Verification items for the finished model (mm, model axes). A direction names the side the tool comes from. Round coordinates to 2 decimals unless told otherwise and drop trailing zeros. Write each loop counter-clockwise with the first axis right and the second up, starting at its lowest first coordinate (ties: lowest second). Pieces come first, ordered by that corner, then holes. Notation, with made-up numbers: (41, -32.5) - (46, -32.5) arc R29 ccw to (46, -6.5) - close; hole circle Ø5 at (44, 28). An arc over 180 degrees is marked (long way). Answer as a JSON object with one key per item and string values.
```python
from build123d import *

# Parameters (mm, degrees)
IZIM1_R                     = 2
IZIM1_R_2                   = 90
Y_KSEKLIK_EKSTR_ZYON1_DEPTH = 3
FILLET1_R                   = 5


with BuildPart() as part:
    # Çizim1 → Yükseklik-Ekstrüzyon1 (new body)
    with BuildSketch(Plane.XY):
        with BuildLine():
            ThreePointArc((81.317279836, -93.817279836), (68.980438262, -79.304237374), (85.290813588, -69.46565423))
            ThreePointArc((85.290813588, -69.46565423), (110, 0), (85.290813588, 69.46565423))
            ThreePointArc((85.290813588, 69.46565423), (68.980438262, 79.304237374), (81.317279836, 93.817279836))
            Line((81.317279836, 93.817279836), (89.317279836, 93.817279836))
            Line((89.317279836, 93.817279836), (89.317279836, 110))
            Line((89.317279836, 110), (-89.317279836, 110))
            Line((-89.317279836, 110), (-89.317279836, 93.817279836))
            Line((-89.317279836, 93.817279836), (-81.317279836, 93.817279836))
            ThreePointArc((-81.317279836, 93.817279836), (-68.980438262, 79.304237374), (-85.290813588, 69.46565423))
            ThreePointArc((-85.290813588, 69.46565423), (-110, 0), (-85.290813588, -69.46565423))
            ThreePointArc((-85.290813588, -69.46565423), (-68.980438262, -79.304237374), (-81.317279836, -93.817279836))
            Line((-81.317279836, -93.817279836), (-89.317279836, -93.817279836))
            Line((-89.317279836, -93.817279836), (-89.317279836, -110))
            Line((-89.317279836, -110), (89.317279836, -110))
            Line((89.317279836, -110), (89.317279836, -93.817279836))
            Line((89.317279836, -93.817279836), (81.317279836, -93.817279836))
        make_face()
        with Locations((-80.9, -101.317279836)):
            Circle(IZIM1_R, mode=Mode.SUBTRACT)
        with Locations((80.9, -101.317279836)):
            Circle(IZIM1_R, mode=Mode.SUBTRACT)
        Circle(IZIM1_R_2, mode=Mode.SUBTRACT)
        with Locations((64.9, 101.317279836)):
            Circle(IZIM1_R, mode=Mode.SUBTRACT)
        with Locations((80.9, 101.317279836)):
            Circle(IZIM1_R, mode=Mode.SUBTRACT)
        with Locations((-80.9, 101.317279836)):
            Circle(IZIM1_R, mode=Mode.SUBTRACT)
        with Locations((-64.9, 101.317279836)):
            Circle(IZIM1_R, mode=Mode.SUBTRACT)
        with Locations((64.9, -101.317279836)):
            Circle(IZIM1_R, mode=Mode.SUBTRACT)
        with Locations((-64.9, -101.317279836)):
            Circle(IZIM1_R, mode=Mode.SUBTRACT)
    extrude(amount=Y_KSEKLIK_EKSTR_ZYON1_DEPTH)

    # Fillet1
    fillet1_edges = [part.edges().sort_by_distance(p)[0] for p in [
        (89.317279836, -93.817279836, 1.5),
        (89.317279836, -110, 1.5),
        (-89.317279836, -110, 1.5),
        (-89.317279836, -93.817279836, 1.5),
        (-85.290813588, -69.46565423, 1.5),
        (-85.290813588, 69.46565423, 1.5),
        (-89.317279836, 93.817279836, 1.5),
        (-89.317279836, 110, 1.5),
        (89.317279836, 110, 1.5),
        (89.317279836, 93.817279836, 1.5),
        (85.290813588, 69.46565423, 1.5),
        (85.290813588, -69.46565423, 1.5),
    ]]
    fillet(fillet1_edges, radius=FILLET1_R)


solid = part.part
```
1. Cross-section at C-C (z = 2.15). Count the separate pieces of the cut face and the enclosed holes in it, plus the area to 3 significant figures.
Completed:
{"separate pieces": "1", "enclosed holes": "9", "area": "15,500 mm^2"}
2. Access from +Z, -Z, +X, -X, +Y, -Y to the whole of each face (thin tool, end or side, straight path). Record for faces 1 (the face through (-87.814, 108.574, 1.521)), 2 (the face through (87.81, -95.24, 1.52)), 3 (the face through (-87.89, 95.32, 1.52)).
Completed:
{"face 1": "+Z, -Z, -X, +Y", "face 2": "+Z, -Z, +X", "face 3": "+Z, -Z, -X"}
3. Cross-section at B-B (y = -43). Record the boundary of the cut face in (x, z), plus the area to 3 significant figures.
Completed:
{"outline": "(-101.25, 0) - (-79.06, 0) - (-79.06, 3) - (-101.25, 3) - close; (79.06, 0) - (101.25, 0) - (101.25, 3) - (79.06, 3) - close", "area": "133 mm^2"}
4. Mould release check, pull along Y, two halves, no side actions. Record for faces 4 (the face through (-87.89, -95.32, 1.52)), 5 (the face through (-82, -40, 0)), 6 (the face through (87.89, -108.5, 1.52)): released by +Y, released by -Y, zero draft, split by the parting line, or undercut.
Completed:
{"face 4": "undercut", "face 5": "zero draft", "face 6": "released by -Y"}
5. Material ranges on probe 1 along Y at (x, z) = (35, 1.2); probe 2 along Y at (x, z) = (3, 1); probe 3 along Y at (x, z) = (-80.9, 0.8), recorded low to high. Write a range as from..to.
Completed:
{"probe 1": "y = -110..-82.92, 82.92..110", "probe 2": "y = -110..-89.95, 89.95..110", "probe 3": "y = -110..-103.32, -99.32..-93.81, -68.82..-39.44, 39.44..68.82, 93.81..99.32, 103.32..110"}
6. Cross-section at A-A (x = 0). Record the boundary of the cut face in (y, z).
Completed:
{"outline": "(-110, 0) - (-90, 0) - (-90, 3) - (-110, 3) - close; (90, 0) - (110, 0) - (110, 3) - (90, 3) - close"}
7. Go/stop test with flat-tipped pins: pin 1 (5 mm diameter, centred on x = -64.9, y = 101.32, fed in from -Z); pin 2 (2.5 mm diameter, centred on x = 80.9, y = -101.32, fed in from +Z). Record where each tip stops, or that it passes through.
Completed:
{"pin 1": "stops at z = 0", "pin 2": "passes through"}
